from build123d import *

# Parameters (mm, degrees)
SKETCH2_W                              = 20
SKETCH2_H                              = 20
BOSS_EXTRUDE1_DEPTH                    = 4
FILLET1_R                              = 2.5
TAPPED_HOLE_FOR_M4X0_7_HELICOIL1_D     = 4.2
TAPPED_HOLE_FOR_M4X0_7_HELICOIL1_DEPTH = 6.8
TAPPED_HOLE_FOR_M4X0_7_HELICOIL1_TIP   = 1.2618073


with BuildPart() as part:
    # Sketch2 → Boss-Extrude1 (new, symmetric)
    with BuildSketch(Plane.XY):
        Rectangle(SKETCH2_W, SKETCH2_H)
    extrude(amount=BOSS_EXTRUDE1_DEPTH, both=True)

    # Fillet1
    fillet1_edges = [part.edges().sort_by_distance(p)[0] for p in [
        (10, 10, 0),
        (10, -10, 0),
    ]]
    fillet(fillet1_edges, radius=FILLET1_R)

    # Tapped Hole for M4x0.7 Helicoil1
    with Locations(Plane.ZY.offset(10)):
        with Locations((0, 5), (0, -5)):
            Hole(TAPPED_HOLE_FOR_M4X0_7_HELICOIL1_D / 2, depth=TAPPED_HOLE_FOR_M4X0_7_HELICOIL1_DEPTH)
            with Locations((0, 0, -(TAPPED_HOLE_FOR_M4X0_7_HELICOIL1_DEPTH + TAPPED_HOLE_FOR_M4X0_7_HELICOIL1_TIP / 2))):  # 118° drill point
                Cone(0, TAPPED_HOLE_FOR_M4X0_7_HELICOIL1_D / 2, TAPPED_HOLE_FOR_M4X0_7_HELICOIL1_TIP, mode=Mode.SUBTRACT)


solid = part.part
Input: part model. Units: mm. Frame: model coordinates. A direction names the side the tool comes from. Give positions to 0.01 mm unless a question says otherwise; leave off trailing zeros. Write each loop counter-clockwise with the first axis right and the second up, starting at its lowest first coordinate (ties: lowest second). Pieces come first, ordered by that corner, then holes. Notation, with made-up numbers: (61.5, 37.5) -> (100.5, 37.5) arc R21 cw to (100.5, 61.5) -> close; hole circle Ø9 at (0, 13). An arc over 180 degrees is marked (long way). Use one line per item in the form item = value. Start each with the question number.
1) Section query A-A on x = -4.25. Return the cut outline in (y, z).
2) Section query B-B on y = 8.75. Return the cut outline in (x, z).
3) Pin query (flat end, axial travel): pin 1 (4 mm diameter, centred on y = -5, z = 0, fed in from -X). Return the tip coordinate at first contact, or that it passes through.
4) Set-up query: faces 4 (the cylindrical face through (-6.55, -7.05, 0.46)), 5 (the flat face through (-10, 0, 0)). Return all of +Z, -Z, +X, -X, +Y, -Y with unobstructed straight access to the full face (end or side cutting, diameter ignored); none if empty.
5) Ray query, probe 1 along Y at (x, z) = (-7.5, 0); probe 2 along Z at (x, y) = (-5.5, 5); probe 3 along Y at (x, z) = (-4, -1.5). Return the intervals inside material, ascending. Write a range as from..to.
6) Draft query along Y for faces 1 (the cylindrical face through (9.287, 9.248, -0.056)), 2 (the conical face through (-2.16, -4.69, 0.2)), 3 (the flat face through (-1, -10, 0)). Return one class per face: pulls with the +Y half, pulls with the -Y half, needs draft (parallel to the pull), parting line crosses it, or undercut.
Outcome:
q1.outline = (-10, -4) -> (10, -4) -> (10, 4) -> (-10, 4) -> close; hole circle Ø4.2 at (-5, 0); hole circle Ø4.2 at (5, 0)
q2.outline = (-10, -4) -> (9.67, -4) -> (9.67, 4) -> (-10, 4) -> close
q3.pin_1 = -3.14
q4.face_4 = -X
q4.face_5 = +Z, -Z, -X, +Y, -Y
q5.probe_1 = -10..-7.1, -2.9..2.9, 7.1..10
q5.probe_2 = -4..-2.1, 2.1..4
q5.probe_3 = -10..-6.47, -3.53..3.53, 6.47..10
q6.face_1 = pulls with the +Y half
q6.face_2 = undercut
q6.face_3 = pulls with the -Y half
